For this review, use the dimensioned drawing (mm, ordinates from the lowest corner) and the shaded views. A direction names the side the tool comes from. Coordinates: 2 decimals unless noted, no trailing zeros. Loops run counter-clockwise (first coordinate to the right, second up) from the corner with the lowest first, then second, coordinate; pieces in that order, holes last. Notation, with made-up numbers: (29.5, 2.25) - (77.5, 2.25) arc R26 ccw to (77.5, 28.25) - close; hole circle Ø3 at (-31, 64). An arc over 180 degrees is marked (long way). Return JSON: item names as keys, results as strings. Group by question number.
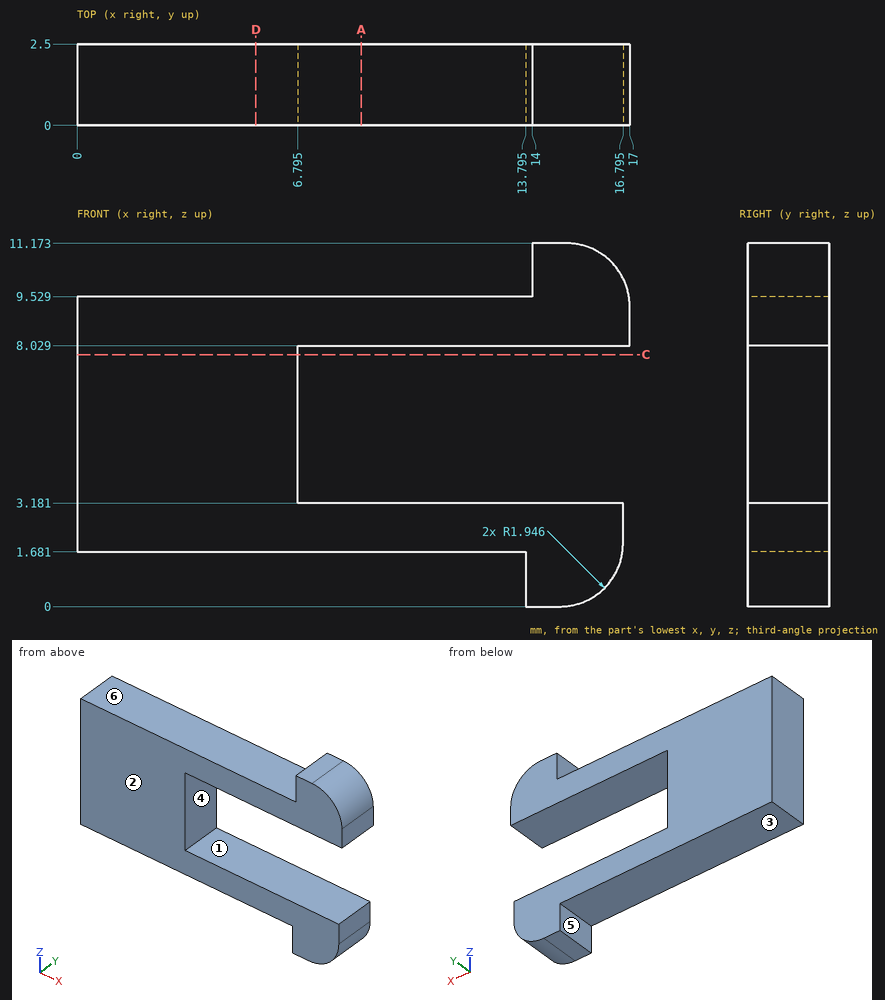
Item 1: To check wall thickness, follow line 1 (Z direction, x = 8, y = 1.7); line 2 (X direction, y = 1.7, z = 5.5) (1 decimal); line 3 (Z direction, x = 5.25, y = 2.3). State the ranges of each line that lie inside material, in increasing order. Write a range as from..to.
Item 2: For the marked faces 1 and 2, list the 3-axis set-ups (+Z, -Z, +X, -X, +Y, -Y) from which the entire face can be reached by the end or side of a thin tool; tool diameter is ignored.
Item 3: Add section A-A (x = 8.75). State the section outline as (y, z) points.
Item 4: Add section C-C (z = 7.75). State the section outline as (x, y) points (1 decimal), then the cut area to 3 significant figures.
Item 5: For P1, Ø1, axis at y = 1.5, z = 3, coming from the +X side (1 decimal); P2, Ø1.3, axis at y = 0.5, z = 1, coming from the -X side (1 decimal); P3, Ø1, axis at x = 4, y = 0.5, coming from the -Z side, all flat-tipped, find the tip position at first contact; note any pin that passes through.
Item 6: Draft analysis for pull direction Z (two halves, no side actions). For the marked faces 3, 4, 5 and 6, state which applies: pulls with the +Z half, pulls with the -Z half, needs draft (parallel to the pull), parting line crosses it, or undercut.
Item 7: Add section D-D (x = 5.5). State the section outline as (y, z) points, then the cut area to 3 significant figures.
Answers below:
{
 "1": {"line 1": "z = 1.68..3.18, 8.03..9.53", "line 2": "x = 0..6.8", "line 3": "z = 1.68..9.53"},
 "2": {"face 1": "+X, +Y, -Y", "face 2": "+Z, -Z, +X, -X, -Y"},
 "3": {"outline": "(0, 1.68) - (2.5, 1.68) - (2.5, 3.18) - (0, 3.18) - close; (0, 8.03) - (2.5, 8.03) - (2.5, 9.53) - (0, 9.53) - close"},
 "4": {"outline": "(0, 0) - (6.8, 0) - (6.8, 2.5) - (0, 2.5) - close", "area": "17.0 mm^2"},
 "5": {"P1": "stops at x = 16.8", "P2": "stops at x = 13.8", "P3": "stops at z = 1.68"},
 "6": {"face 3": "pulls with the -Z half", "face 4": "undercut", "face 5": "needs draft", "face 6": "pulls with the +Z half"},
 "7": {"outline": "(0, 1.68) - (2.5, 1.68) - (2.5, 9.53) - (0, 9.53) - close", "area": "19.6 mm^2"}
}
